Here's how the part is built. I have some questions about the finished solid (model axes, mm). A direction names the side the tool comes from. Give positions to 0.01 mm unless a question says otherwise; leave off trailing zeros. Loops run counter-clockwise (first coordinate to the right, second up) from the corner with the lowest first, then second, coordinate; pieces in that order, holes last.
Q1. Thinking about a two-plate mould opening in Z: for faces 5 (the face through (-1, -15, -43.1)), 6 (the face through (-1, -17, 45.1)), 7 (the face through (50.67, -13.24, -43.6)), which applies, pulls with the +Z half, pulls with the -Z half, needs draft (parallel to the pull), parting line crosses it, or undercut?
Q2. I'm going to push a flat-ended pin straight in: P1, Ø12, axis at x = -18.5, z = 17.5, coming from the -Y side. Where does the tip first touch, or does it pass through?
Q3. Suppose I cut it at A-A (x = 35). List the corners of the cut face in (y, z) for me.
Q4. I need wall thicknesses on probe 1 along Z at (x, y) = (-43.5, -4); probe 2 along X at (y, z) = (-23, -27); probe 3 along Z at (x, y) = (-20, -34). Which ranges of each line are inside material? Lowest first, please.
Q5. For faces 1 (the face through (-1, -35, 43.3)), 2 (the face through (-50.1, -15, -1)), 3 (the face through (-50.3, -35, -25)), 4 (the face through (0.673, -31.922, -44.197)), which set-ups out of +Z, -Z, +X, -X, +Y, -Y let a thin tool reach every point of the face, with its end or its side?
Q6. Suppose I cut it at D-D (z = -6). List the corners of the cut face in (x, y) for me, and give its area (3 significant figures).
Q7. Suppose I cut it at C-C (y = -18). List the corners of the cut face in (x, z) for me, and give its area (3 significant figures).
Q8. Suppose I cut it at B-B (z = 34.5). List the corners of the cut face in (x, y) for me, and give its area (3 significant figures).
```python
from build123d import *

# Parameters (mm, degrees)
ESQUISSE1_W              = 104.2
ESQUISSE1_H              = 90.2
BOSS_EXTRU_1_DEPTH       = 2
ESQUISSE2_W              = 104.2
ESQUISSE2_H              = 90.2
ESQUISSE2_W_2            = 100.2
ESQUISSE2_H_2            = 86.2
BOSS_EXTRU_2_DEPTH       = 36.5
ENL_V_MAT_EXTRU_1_DEPTH  = 12
SYM_TRIE2_COPY_1_DEPTH   = 12
CONG_3_R                 = 1
CONG_1_R                 = 5
ENL_V_MAT_EXTRU_2_DEPTH  = 78.978650924
ENL_V_MAT_EXTRU_3_DEPTH  = 78.978651027
ESQUISSE15_W             = 100.6
ESQUISSE15_H             = 86.6
ENL_V_MAT_EXTRU_10_DEPTH = 4.5
ENL_V_MAT_EXTRU_11_REACH = 121.264
ESQUISSE17_W             = 14
ESQUISSE17_H             = 9
CONG_4_R                 = 1


with BuildPart() as part:
    # Esquisse1 → Boss.-Extru.1 (new body)
    with BuildSketch(Plane(origin=(0, 0, 0), x_dir=(1, 0, 0), z_dir=(0, 1, 0))):
        Rectangle(ESQUISSE1_W, ESQUISSE1_H)
    extrude(amount=BOSS_EXTRU_1_DEPTH)

    # Esquisse2 → Boss.-Extru.2 (add)
    with BuildSketch(Plane.XZ):
        Rectangle(ESQUISSE2_W, ESQUISSE2_H)
        Rectangle(ESQUISSE2_W_2, ESQUISSE2_H_2, mode=Mode.SUBTRACT)
    extrude(amount=BOSS_EXTRU_2_DEPTH)

    # Esquisse3 → Enlèv. mat.-Extru.1 (cut)
    with BuildSketch(Plane.XZ.offset(36.5)):
        Polygon((-50.1, 41.1), (-50.1, 43.1), (-48.1, 43.1), (-48.1, 45.1), (-52.1, 45.1), (-52.1, 41.1), align=None)
    enl_v_mat_extru_1 = extrude(amount=-ENL_V_MAT_EXTRU_1_DEPTH, mode=Mode.SUBTRACT)

    # Symétrie1: Enlèv. mat.-Extru.1 across plane
    add(enl_v_mat_extru_1.mirror(Plane.XY), mode=Mode.SUBTRACT)

    # Symétrie2: Enlèv. mat.-Extru.1 across plane
    add(enl_v_mat_extru_1.mirror(Plane(origin=(0, 0, 0), x_dir=(0, 0, 1), z_dir=(1, 0, 0))), mode=Mode.SUBTRACT)

    # Symétrie2 copy 1 sketch → Symétrie2 copy 1 (cut)
    with BuildSketch(Plane(origin=(0, -36.5, 0), x_dir=(-1, 0, 0), z_dir=(0, -1, 0))):
        Polygon((-50.1, 41.1), (-50.1, 43.1), (-48.1, 43.1), (-48.1, 45.1), (-52.1, 45.1), (-52.1, 41.1), align=None)
    extrude(amount=-SYM_TRIE2_COPY_1_DEPTH, mode=Mode.SUBTRACT)

    # Congé3
    cong_3_edges = [part.edges().sort_by_distance(p)[0] for p in [
        (-48.1, -30.5, 45.1),
        (-48.1, -30.5, 43.1),
        (-50.1, -30.5, 41.1),
        (-52.1, -30.5, 41.1),
        (48.1, -30.5, 45.1),
        (48.1, -30.5, 43.1),
        (52.1, -30.5, 41.1),
        (50.1, -30.5, 41.1),
        (52.1, -30.5, -41.1),
        (50.1, -30.5, -41.1),
        (48.1, -30.5, -43.1),
        (48.1, -30.5, -45.1),
        (-48.1, -30.5, -45.1),
        (-48.1, -30.5, -43.1),
        (-50.1, -30.5, -41.1),
        (-52.1, -30.5, -41.1),
    ]]
    fillet(cong_3_edges, radius=CONG_3_R - 0.0001)  # a hair under: the kernel refuses the full size

    # Congé1
    cong_1_edges = [part.edges().sort_by_distance(p)[0] for p in [
        (52.1, -11.25, 45.1),
        (52.1, -11.25, -45.1),
        (-52.1, -11.25, -45.1),
        (-52.1, -11.25, 45.1),
    ]]
    fillet(cong_1_edges, radius=CONG_1_R)

    # Esquisse4 → Enlèv. mat.-Extru.2 (cut, symmetric)
    with BuildSketch(Plane(origin=(0, 0, 0), x_dir=(0, 0, -1), z_dir=(1, 0, 0))):
        with BuildLine():
            Line((-43.1, -30.9), (-43.1, -33.1))
            ThreePointArc((-43.1, -33.1), (-44.2, -32), (-43.1, -30.9))
        make_face()
    enl_v_mat_extru_2 = extrude(amount=ENL_V_MAT_EXTRU_2_DEPTH, both=True, mode=Mode.SUBTRACT)

    # Symétrie4: Enlèv. mat.-Extru.2 across plane
    add(enl_v_mat_extru_2.mirror(Plane.XY), mode=Mode.SUBTRACT)

    # Esquisse5 → Enlèv. mat.-Extru.3 (cut, symmetric)
    with BuildSketch(Plane.XY):
        with BuildLine():
            Line((-50.1, -30.9), (-50.1, -33.1))
            ThreePointArc((-50.1, -33.1), (-51.2, -32), (-50.1, -30.9))
        make_face()
    enl_v_mat_extru_3 = extrude(amount=ENL_V_MAT_EXTRU_3_DEPTH, both=True, mode=Mode.SUBTRACT)

    # Symétrie5: Enlèv. mat.-Extru.3 across plane
    add(enl_v_mat_extru_3.mirror(Plane(origin=(0, 0, 0), x_dir=(0, 0, 1), z_dir=(1, 0, 0))), mode=Mode.SUBTRACT)

    # Esquisse15 → Enlèv. mat.-Extru.10 (cut)
    with BuildSketch(Plane.XZ.offset(36.5)):
        Rectangle(ESQUISSE15_W, ESQUISSE15_H)
    extrude(amount=-ENL_V_MAT_EXTRU_10_DEPTH, mode=Mode.SUBTRACT)

    # Enlèv. mat.-Extru.11: up to this face of the body (flat: up to its plane)
    enl_v_mat_extru_11_end = Plane(part.part.faces().sort_by_distance((-50.1, -15.270818347, 0))[0])
    # Esquisse17 → Enlèv. mat.-Extru.11 (cut, up to the picked face)
    with BuildSketch(Plane.ZY.offset(52.1), mode=Mode.PRIVATE) as enl_v_mat_extru_11_sk1:
        with Locations((-2.74, -36.5)):
            Rectangle(ESQUISSE17_W, ESQUISSE17_H)
    enl_v_mat_extru_11_tool1 = split(extrude(enl_v_mat_extru_11_sk1.sketch, amount=-ENL_V_MAT_EXTRU_11_REACH, mode=Mode.PRIVATE), bisect_by=enl_v_mat_extru_11_end, keep=Keep.BOTH, mode=Mode.PRIVATE)
    add(enl_v_mat_extru_11_tool1.solids().sort_by(Axis((-52.1, -36.5, -2.74), (1, 0, 0)))[0], mode=Mode.SUBTRACT)

    # Congé4
    cong_4_edges = [part.edges().sort_by_distance(p)[0] for p in [
        (-51.65, -32, -9.74),
        (-51.65, -32, 4.26),
    ]]
    fillet(cong_4_edges, radius=CONG_4_R)


solid = part.part
```
Solutions:
1. face 5: undercut
1. face 6: pulls with the +Z half
1. face 7: pulls with the -Z half
2. P1: stops at y = 0
3. outline: (-36.5, -45.1) - (2, -45.1) - (2, 45.1) - (-36.5, 45.1) - (-36.5, 43.3) - (-33.08, 43.3) arc R1.1 cw to (-30.9, 43.1) - (0, 43.1) - (0, -43.1) - (-30.9, -43.1) arc R1.1 cw to (-33.08, -43.3) - (-36.5, -43.3) - close
4. probe 1: z = -45.1 to -43.1, 43.1 to 45.1
4. probe 2: x = -52.1 to -50.1, 50.1 to 52.1
4. probe 3: z = -45.1 to -43.3, 43.3 to 45.1
5. face 1: +X, -X, -Y
5. face 2: -Y
5. face 3: +Z, -Z, -Y
5. face 4: +X, -X
6. outline: (-52.1, -32) - (-51.2, -32) arc R1.1 cw to (-50.1, -30.9) - (-50.1, 0) - (50.1, 0) - (50.1, -30.9) arc R1.1 cw to (50.3, -33.08) - (50.3, -36.5) - (52.1, -36.5) - (52.1, 2) - (-52.1, 2) - close
6. area: 342 mm2
7. outline: (-52.1, -40.1) arc R5 ccw to (-47.1, -45.1) - (47.1, -45.1) arc R5 ccw to (52.1, -40.1) - (52.1, 40.1) arc R5 ccw to (47.1, 45.1) - (-47.1, 45.1) arc R5 ccw to (-52.1, 40.1) - close; hole (-50.1, -43.1) - (50.1, -43.1) - (50.1, 43.1) - (-50.1, 43.1) - close
7. area: 740 mm2
8. outline: (-52.1, -36.5) - (-50.3, -36.5) - (-50.3, -33.08) arc R1.1 cw to (-50.1, -30.9) - (-50.1, 0) - (50.1, 0) - (50.1, -30.9) arc R1.1 cw to (50.3, -33.08) - (50.3, -36.5) - (52.1, -36.5) - (52.1, 2) - (-52.1, 2) - close
8. area: 349 mm2
